Verification items for the finished model (mm, model axes). Face numbers are marked on the shaded views. A direction names the side the tool comes from. Coordinates: 2 decimals unless noted, no trailing zeros. Write each loop counter-clockwise with the first axis right and the second up, starting at its lowest first coordinate (ties: lowest second). Pieces come first, ordered by that corner, then holes. Notation, with made-up numbers: (57, 84) -> (69, 84) arc R14 ccw to (69, 111) -> close; hole circle Ø5 at (-27, 61). An arc over 180 degrees is marked (long way). Answer in a Markdown table with one row per item.
```python
from build123d import *

# Parameters (mm, degrees)
SKETCH_1_W          = 16
SKETCH_1_H          = 11
EXTRUDE_1_DEPTH     = 2
EXTRUDE_START       = 2
EXTRUDE_2_DEPTH     = 6
SKETCH_3_W          = 3.5
SKETCH_3_H          = 6
CUT_EXTRUDE_1_DEPTH = 13.267844146


with BuildPart() as part:
    # 草图1 → 凸台-拉伸1 (new body)
    with BuildSketch(Plane(origin=(0, 0, 0), x_dir=(1, 0, 0), z_dir=(0, 1, 0))):
        Rectangle(SKETCH_1_W, SKETCH_1_H)
    extrude(amount=EXTRUDE_1_DEPTH)

    # 草图2 → 凸台-拉伸2 (add)
    with BuildSketch(Plane(origin=(0, 0, 0), x_dir=(0, 0, -1), z_dir=(1, 0, 0)).offset(EXTRUDE_START)):
        with BuildLine():
            Line((-5.5, 2), (-4.75, 2))
            ThreePointArc((-4.75, 2), (0, 6.75), (4.75, 2))
            Line((4.75, 2), (5.5, 2))
            ThreePointArc((5.5, 2), (0, 7.5), (-5.5, 2))
        make_face()
    extrude(amount=EXTRUDE_2_DEPTH)

    # 草图3 → 切除-拉伸1 (cut, through all)
    with BuildSketch(Plane.XZ):
        Rectangle(SKETCH_3_W, SKETCH_3_H)
    extrude(amount=-CUT_EXTRUDE_1_DEPTH, mode=Mode.SUBTRACT)


solid = part.part
```
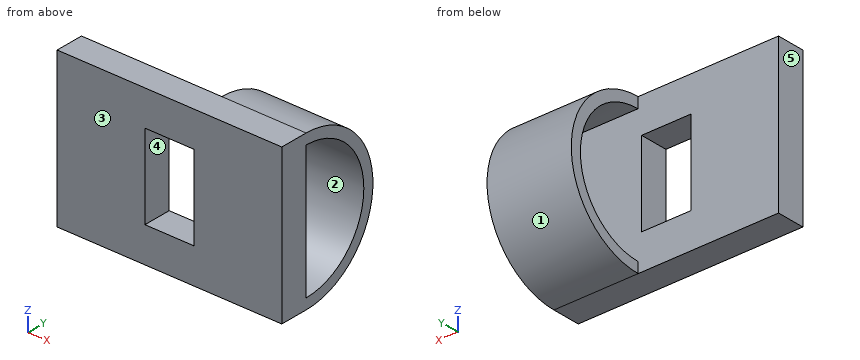
1. Tool access check on the marked faces 4 and 5. Record the directions out of +Z, -Z, +X, -X, +Y, -Y that give a thin tool (end or side, any length) a straight path to the whole face; none if there is none.
Geometry says:
| item | result |
|---|---|
| face 4 | +Y, -Y |
| face 5 | +Z, -Z, -X, +Y, -Y |
2. Section check C-C, the plane y = 4.5. Record the boundary of the cut face in (x, z), plus the area to 3 significant figures.
Geometry says:
| item | result |
|---|---|
| outline | (2, -4.9) -> (8, -4.9) -> (8, -4.04) -> (2, -4.04) -> close; (2, 4.04) -> (8, 4.04) -> (8, 4.9) -> (2, 4.9) -> close |
| area | 10.3 mm^2 |
3. Thickness scan on line 1 (Z direction, x = -0.5, y = 1); line 2 (Y direction, x = -0.75, z = -4); line 3 (Z direction, x = 3.75, y = 3.5). Record the ranges inside material, lowest first. Write a range as from..to.
Geometry says:
| item | result |
|---|---|
| line 1 | -5.5..-3, 3..5.5 |
| line 2 | 0..2 |
| line 3 | -5.29..-4.51, 4.51..5.29 |
4. Depth check by flat-ended pin: P1, Ø3, axis at y = 4.5, z = -2, coming from the +X side; P2, Ø6, axis at x = 6, z = -4, coming from the +Y side. Enter the tip coordinate at first touch or a pass-through.
Geometry says:
| item | result |
|---|---|
| P1 | through |
| P2 | y = 7.41 |
5. Section check B-B, the plane z = 0. Record the boundary of the cut face in (x, y), plus the area to 3 significant figures.
Geometry says:
| item | result |
|---|---|
| outline | (-8, 0) -> (-1.75, 0) -> (-1.75, 2) -> (-8, 2) -> close; (1.75, 0) -> (8, 0) -> (8, 2) -> (1.75, 2) -> close; (2, 6.75) -> (8, 6.75) -> (8, 7.5) -> (2, 7.5) -> close |
| area | 29.5 mm^2 |
6. Mould release check, pull along Z, two halves, no side actions. Record for the marked faces 1, 2 and 3: released by +Z, released by -Z, zero draft, split by the parting line, or undercut.
Geometry says:
| item | result |
|---|---|
| face 1 | split by the parting line |
| face 2 | undercut |
| face 3 | zero draft |
7. Section check D-D, the plane x = 5.75. Record the boundary of the cut face in (y, z), plus the area to 3 significant figures.
Geometry says:
| item | result |
|---|---|
| outline | (0, -5.5) -> (2, -5.5) arc R5.5 ccw to (2, 5.5) -> (0, 5.5) -> close; hole (2, -4.75) arc R4.75 ccw to (2, 4.75) -> close |
| area | 34.1 mm^2 |
8. Section check A-A, the plane x = 1.5. Record the boundary of the cut face in (y, z), plus the area to 3 significant figures.
Geometry says:
| item | result |
|---|---|
| outline | (0, -5.5) -> (2, -5.5) -> (2, -3) -> (0, -3) -> close; (0, 3) -> (2, 3) -> (2, 5.5) -> (0, 5.5) -> close |
| area | 10.0 mm^2 |
